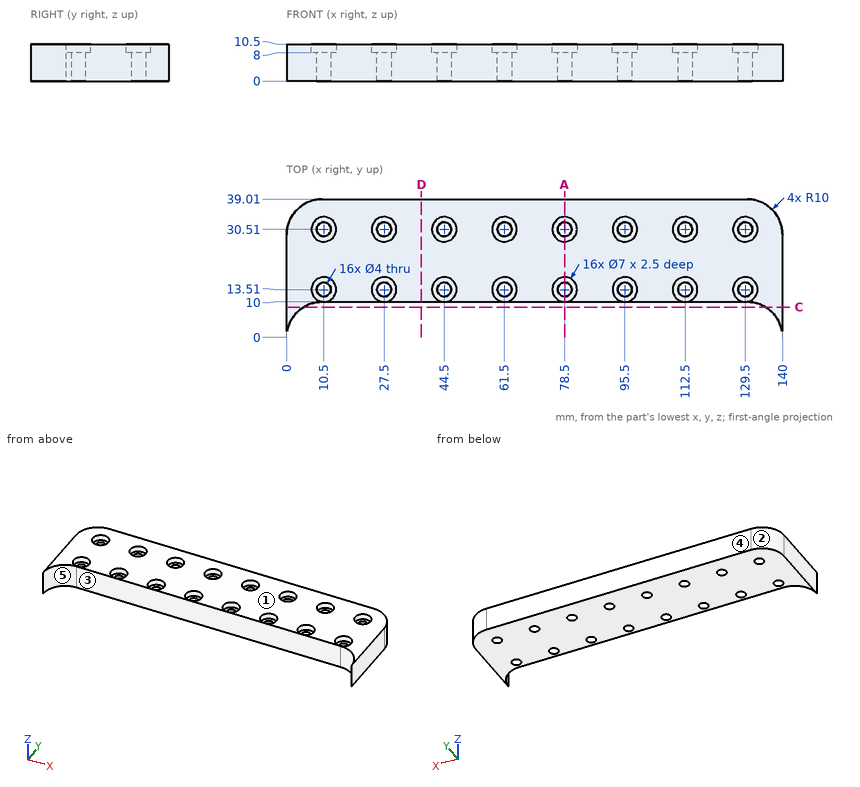
Verification items for this drawing (mm, ordinates from the low corner). A direction names the side the tool comes from. Round coordinates to 2 decimals unless told otherwise and drop trailing zeros. Loops run counter-clockwise (first coordinate to the right, second up) from the corner with the lowest first, then second, coordinate; pieces in that order, holes last. Notation, with made-up numbers: (-11.5, 57) - (46.5, 57) arc R21 cw to (46.5, 64) - close; hole circle Ø11 at (81.25, 36.5). An arc over 180 degrees is marked (long way). Write item = value, one per line.
Q1. Mould release check, pull along X, two halves, no side actions. Record for the marked faces 1, 2 and 3: +X half, -X half, draft (parallel to the pull), parting line (faces both ways), or undercut.
Here are the results:
face_1 = draft
face_2 = -X half
face_3 = undercut
Q2. Sectioned sample at A-A on x = 78.5. State how many separate pieces and enclosed holes the cut face has, plus the area to 3 significant figures.
Here are the results:
separate_pieces = 3
enclosed_holes = 0
area = 206 mm^2
Q3. Material ranges on L1, parallel to Y at x = 61.5, z = 3.75; L2, parallel to Y at x = 116.5, z = 9; L3, parallel to X at y = 6.5, z = 5.75, recorded low to high.
Here are the results:
L1 = 10 to 11.51, 15.51 to 28.51, 32.51 to 39.01
L2 = 10 to 39.01
L3 = 0 to 2.4, 137.6 to 140
Q4. Sectioned sample at C-C on y = 8.5. Record the boundary of the cut face in (x, z), plus the area to 3 significant figures.
Here are the results:
outline = (0, 0) - (4.73, 0) - (4.73, 10.5) - (0, 10.5) - close; (135.27, 0) - (140, 0) - (140, 10.5) - (135.27, 10.5) - close
area = 99.4 mm^2
Q5. Tool access check on the marked faces 4 and 5. Record the directions out of +Z, -Z, +X, -X, +Y, -Y that give a thin tool (end or side, any length) a straight path to the whole face; none if there is none.
Here are the results:
face_4 = +Z, -Z, +X, -X, +Y
face_5 = +Z, -Z, -Y
Q6. Sectioned sample at D-D on x = 38. Record the boundary of the cut face in (y, z).
Here are the results:
outline = (10, 0) - (39.01, 0) - (39.01, 10.5) - (10, 10.5) - close
Q7. Depth check by flat-ended pin: pin 1 (2.5 mm diameter, centred on x = 78.5, y = 13.51, fed in from +Z); pin 2 (6.5 mm diameter, centred on x = 95.5, y = 13.51, fed in from +Z). Enter the tip coordinate at first touch or a pass-through.
Here are the results:
pin_1 = through
pin_2 = 8
